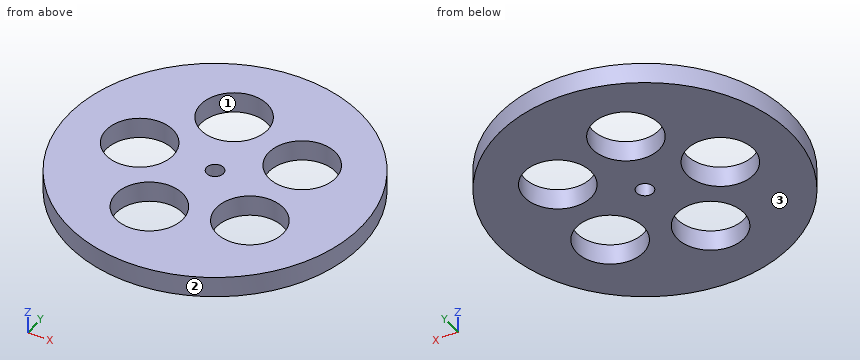
from build123d import *

# Parameters (mm, degrees)
ESQUISSE1_R             = 35
ESQUISSE1_R_2           = 2
CIRCONFERENCE_DEPTH     = 5
ESQUISSE2_R             = 8
ENL_V_MAT_EXTRU_1_DEPTH = 6


with BuildPart() as part:
    # Esquisse1 → circonference (new body)
    with BuildSketch(Plane.XY):
        Circle(ESQUISSE1_R)
        Circle(ESQUISSE1_R_2, mode=Mode.SUBTRACT)
    extrude(amount=CIRCONFERENCE_DEPTH)

    # Esquisse2 → Enlèv. mat.-Extru.1 (cut, through all)
    with BuildSketch(Plane.XY.offset(5)):
        with Locations((-17.810269486, 0)):
            Circle(ESQUISSE2_R)
        with Locations((-5.503675945, 16.938572851)):
            Circle(ESQUISSE2_R)
        with Locations((14.408810688, 10.468613743)):
            Circle(ESQUISSE2_R)
        with Locations((14.408810688, -10.468613743)):
            Circle(ESQUISSE2_R)
        with Locations((-5.503675945, -16.938572851)):
            Circle(ESQUISSE2_R)
    extrude(amount=-ENL_V_MAT_EXTRU_1_DEPTH, mode=Mode.SUBTRACT)


solid = part.part
Verification items for the finished model (mm, model axes). Face numbers are marked on the shaded views. Round coordinates to 2 decimals unless told otherwise and drop trailing zeros. Loops run counter-clockwise (first coordinate to the right, second up) from the corner with the lowest first, then second, coordinate; pieces in that order, holes last. Notation, with made-up numbers: (57.25, -3) - (105.25, -3) arc R27 cw to (105.25, 24) - close; hole circle Ø7 at (-38.75, 3.5). An arc over 180 degrees is marked (long way). Use a Markdown table: item, result. Add a question column.
1. Section check B-B, the plane x = -8. Record the boundary of the cut face in (y, z).
2. Gauge pin test, flat ends, axial feed: pin 1 (6 mm diameter, centred on x = -14.5, y = -9, fed in from -Z); pin 2 (1 mm diameter, centred on x = -1, z = 2, fed in from -Y); pin 3 (1.5 mm diameter, centred on y = 18.5, z = 2, fed in from +X); pin 4 (2 mm diameter, centred on x = 24.5, z = 4, fed in from +Y). Record the tip position at first contact, or that the pin passes through.
3. Section check D-D, the plane x = 0. Record the boundary of the cut face in (y, z).
4. Thickness scan on probe 1 along Y at (x, z) = (0, 1.4); probe 2 along Y at (x, z) = (10.5, 4.35); probe 3 along X at (y, z) = (-5, 1.7). Record the ranges inside material, lowest first. Write a range as [from, to].
5. Section check C-C, the plane y = 20. Record the boundary of the cut face in (x, z).
6. Release check for a two-part mould opening along X. For the marked faces 1, 2 and 3 record: released by +X, released by -X, zero draft, split by the parting line, or undercut.
7. Section check A-A, the plane y = 0. Record the boundary of the cut face in (x, z).
Checks:
| question | item | result |
|---|---|---|
| 1 | outline | (-34.07, 0) - (-24.54, 0) - (-24.54, 5) - (-34.07, 5) - close; (-9.34, 0) - (9.34, 0) - (9.34, 5) - (-9.34, 5) - close; (24.54, 0) - (34.07, 0) - (34.07, 5) - (24.54, 5) - close |
| 2 | pin 1 | stops at z = 0 |
| 2 | pin 2 | stops at y = -35 |
| 2 | pin 3 | stops at x = 30.17 |
| 2 | pin 4 | stops at y = 25.94 |
| 3 | outline | (-35, 0) - (-22.74, 0) - (-22.74, 5) - (-35, 5) - close; (-11.13, 0) - (-2, 0) - (-2, 5) - (-11.13, 5) - close; (2, 0) - (11.13, 0) - (11.13, 5) - (2, 5) - close; (22.74, 0) - (35, 0) - (35, 5) - (22.74, 5) - close |
| 4 | probe 1 | y = [-35, -22.74], [-11.13, -2], [2, 11.13], [22.74, 35] |
| 4 | probe 2 | y = [-33.39, -17.45], [-3.49, 3.49], [17.45, 33.39] |
| 4 | probe 3 | x = [-34.64, -24.06], [-11.57, 8.57], [20.25, 34.64] |
| 5 | outline | (-28.72, 0) - (-12.89, 0) - (-12.89, 5) - (-28.72, 5) - close; (1.89, 0) - (28.72, 0) - (28.72, 5) - (1.89, 5) - close |
| 6 | face 1 | undercut |
| 6 | face 2 | split by the parting line |
| 6 | face 3 | zero draft |
| 7 | outline | (-35, 0) - (-25.81, 0) - (-25.81, 5) - (-35, 5) - close; (-9.81, 0) - (-2, 0) - (-2, 5) - (-9.81, 5) - close; (2, 0) - (35, 0) - (35, 5) - (2, 5) - close |
